Geometry check sheet. Reference: the model listing, model coordinates, mm. A direction names the side the tool comes from. Give positions to 0.01 mm unless a question says otherwise; leave off trailing zeros. Loops run counter-clockwise (first coordinate to the right, second up) from the corner with the lowest first, then second, coordinate; pieces in that order, holes last. Notation, with made-up numbers: (-2.75, 19.5) -> (25.25, 19.5) arc R19 ccw to (25.25, 30.5) -> close; hole circle Ø7 at (-22, 46). An arc over 180 degrees is marked (long way). Answer as a JSON object with one key per item and string values.
from build123d import *

# Parameters (mm, degrees)
F0_R     = 16
F0_R_2   = 9.5
F1_DEPTH = 2
F3_DEPTH = 10


with BuildPart() as f1:
    # F0 (on Front) → F1 (new body)
    with BuildSketch(Plane.XZ):
        Circle(F0_R)
        Circle(F0_R_2, mode=Mode.SUBTRACT)
    extrude(amount=F1_DEPTH)

    # F2 (on Front) → F3 (join)
    with BuildSketch(Plane.XZ):
        with BuildLine():
            ThreePointArc((9.075132, -5.281286), (10.499984, -0.018081), (9.093267, 5.25))
            ThreePointArc((9.093267, 5.25), (0, 10.5), (-9.093267, 5.25))
            ThreePointArc((-9.093267, 5.25), (-10.5, 0), (-9.093267, -5.25))
            ThreePointArc((-9.093267, -5.25), (-0.018081, -10.499984), (9.075132, -5.281286))
        make_face()
        with BuildLine():
            ThreePointArc((-7.413502, -5.35), (-9.142347, 0), (-7.413502, 5.35))
            Line((-7.413502, 5.35), (7.420145, 5.35))
            ThreePointArc((7.420145, 5.35), (9.147735, 0), (7.420145, -5.35))
            Line((7.420145, -5.35), (-7.413502, -5.35))
        make_face(mode=Mode.SUBTRACT)
    extrude(amount=F3_DEPTH)


solid = f1.part
1) Section check B-B on x = 0. Record the cut outline in (y, z).
Geometry check:
{"outline": "(-10, -10.5) -> (-2, -10.5) -> (-2, -16) -> (0, -16) -> (0, -5.35) -> (-10, -5.35) -> close; (-10, 5.35) -> (0, 5.35) -> (0, 16) -> (-2, 16) -> (-2, 10.5) -> (-10, 10.5) -> close"}
2) Draft check along Z on faces 4 (the face through (0, -10, -7)), 5 (the face through (-3.47, -0.99, -15.62)), 6 (the face through (0, -5, 5.35)). Enter one of: pulls with the +Z half, pulls with the -Z half, needs draft (parallel to the pull), parting line crosses it, or undercut.
Geometry check:
{"face 4": "needs draft", "face 5": "parting line crosses it", "face 6": "undercut"}
3) Tool access check on faces 1 (the face through (0, 0, -7)), 2 (the face through (10.4, -2, -3.3)), 3 (the face through (0, -5, -5.35)). Record the directions out of +Z, -Z, +X, -X, +Y, -Y that give a thin tool (end or side, any length) a straight path to the whole face; none if there is none.
Geometry check:
{"face 1": "+Z, -Z, +X, -X, +Y", "face 2": "-Y", "face 3": "+Y, -Y"}
4) Section check D-D on y = -1.25. Record the cut outline in (x, z), plus the area to 3 significant figures.
Geometry check:
{"outline": "circle Ø32 at (0, 0); hole (-7.41, -5.35) -> (7.42, -5.35) arc R9.15 ccw to (7.42, 5.35) -> (-7.41, 5.35) arc R9.14 ccw to start", "area": "620 mm2"}
5) Material ranges on line 1 along X through (y, z) = (-6.5, -2.5); line 2 along Y through (x, z) = (6.5, 13.5); line 3 along Z through (x, y) = (1, -6.25), recorded low to high. Write a range as from..to.
Geometry check:
{"line 1": "x = -10.2..-8.79, 8.8..10.2", "line 2": "y = -2..0", "line 3": "z = -10.45..-5.35, 5.35..10.45"}
6) Section check A-A on z = 0. Record the cut outline in (x, y).
Geometry check:
{"outline": "(-16, -2) -> (-10.5, -2) -> (-10.5, -10) -> (-9.14, -10) -> (-9.14, 0) -> (-16, 0) -> close; (9.15, -10) -> (10.5, -10) -> (10.5, -2) -> (16, -2) -> (16, 0) -> (9.15, 0) -> close"}
7) Depth check by flat-ended pin: P1, Ø2, axis at x = -10, y = -5, coming from the -Z side; P2, Ø4, axis at x = -10, z = -9.5, coming from the -Y side; P3, Ø3, axis at x = -9.5, y = -9, coming from the -Z side. Enter the tip coordinate at first touch or a pass-through.
Geometry check:
{"P1": "stops at z = -5.41", "P2": "stops at y = -2", "P3": "stops at z = -6.8"}
8) Section check C-C on y = -5. Record the cut outline in (x, z).
Geometry check:
{"outline": "(-9.09, -5.25) arc R10.5 ccw to (9.08, -5.28) arc R10.5 ccw to (9.09, 5.25) arc R10.5 ccw to (-9.09, 5.25) arc R10.5 ccw to start; hole (-7.41, -5.35) -> (7.42, -5.35) arc R9.15 ccw to (7.42, 5.35) -> (-7.41, 5.35) arc R9.14 ccw to start"}
